from build123d import *

# Parameters (mm, degrees)
SKETCH_W        = 49
SKETCH_H        = 40
PAD_DEPTH       = 33
SKETCH001_W     = 47
SKETCH001_H     = 21
POCKET_DEPTH    = 31
SKETCH002_W     = 42
SKETCH002_H     = 19
POCKET001_DEPTH = 31
SKETCH003_W     = 7
SKETCH003_H     = 7
POCKET002_DEPTH = 31
SKETCH004_W     = 10
SKETCH004_H     = 10
PAD001_DEPTH    = 27
SKETCH005_W     = 10
SKETCH005_H     = 8
POCKET003_DEPTH = 27
SKETCH006_W     = 7
SKETCH006_H     = 12
POCKET004_DEPTH = 4
SKETCH007_W     = 5
SKETCH007_H     = 10
POCKET005_DEPTH = 27
FILLET_R        = 4
SKETCH008_R     = 1.6
POCKET006_DEPTH = 6.001
SKETCH009_R     = 1.6
POCKET007_DEPTH = 6.001
SKETCH010_R     = 2.75
POCKET008_DEPTH = 27
FILLET001_R     = 2
FILLET002_R     = 4
SKETCH011_W     = 11.5
SKETCH011_H     = 8.5
PAD002_DEPTH    = 2
FILLET003_R     = 2
FILLET004_R     = 4
FILLET005_R     = 6
FILLET006_R     = 2
FILLET007_R     = 2


with BuildPart() as part:
    # Sketch → Pad (new body)
    with BuildSketch(Plane.XY):
        with Locations((24.5, 20)):
            Rectangle(SKETCH_W, SKETCH_H)
    extrude(amount=PAD_DEPTH)

    # Sketch001 → Pocket (cut)
    with BuildSketch(Plane.XY):
        with Locations((23.5, 10.5)):
            Rectangle(SKETCH001_W, SKETCH001_H)
    extrude(amount=POCKET_DEPTH, mode=Mode.SUBTRACT)

    # Sketch002 (on Face4 of Pocket) → Pocket001 (cut)
    with BuildSketch(Plane(origin=(0, 0, 0), x_dir=(1, 0, 0), z_dir=(0, 0, -1))):
        with Locations((28, -30.5)):
            Rectangle(SKETCH002_W, SKETCH002_H)
    extrude(amount=-POCKET001_DEPTH, mode=Mode.SUBTRACT)

    # Sketch003 (on Face10 of Pocket001) → Pocket002 (cut)
    with BuildSketch(Plane(origin=(0, 0, 0), x_dir=(1, 0, 0), z_dir=(0, 0, -1))):
        with Locations((3.5, -24.5)):
            Rectangle(SKETCH003_W, SKETCH003_H)
    extrude(amount=-POCKET002_DEPTH, mode=Mode.SUBTRACT)

    # Sketch004 (on Face12 of Pocket002) → Pad001 (join)
    with BuildSketch(Plane(origin=(0, 0, 31), x_dir=(1, 0, 0), z_dir=(0, 0, -1))):
        with Locations((42, -5)):
            Rectangle(SKETCH004_W, SKETCH004_H)
    extrude(amount=PAD001_DEPTH)

    # Sketch005 (on Face7 of Pad001) → Pocket003 (cut)
    with BuildSketch(Plane.XY.offset(33)):
        with Locations((44, 4)):
            Rectangle(SKETCH005_W, SKETCH005_H)
    extrude(amount=-POCKET003_DEPTH, mode=Mode.SUBTRACT)

    # Sketch006 (on Face2 of Pocket003) → Pocket004 (cut)
    with BuildSketch(Plane(origin=(0, 0, 0), x_dir=(1, 0, 0), z_dir=(0, 0, -1))):
        with Locations((3.5, -34)):
            Rectangle(SKETCH006_W, SKETCH006_H)
    extrude(amount=-POCKET004_DEPTH, mode=Mode.SUBTRACT)

    # Sketch007 (on Face7 of Pocket004) → Pocket005 (cut)
    with BuildSketch(Plane.XY.offset(33)):
        with Locations((2.5, 35)):
            Rectangle(SKETCH007_W, SKETCH007_H)
    extrude(amount=-POCKET005_DEPTH, mode=Mode.SUBTRACT)

    # Fillet
    fillet_edges = [part.edges().sort_by_distance(p)[0] for p in [
        (39, 8, 19.5),
    ]]
    fillet(fillet_edges, radius=FILLET_R)

    # Sketch008 (on Face11 of Fillet) → Pocket006 (cut, through all)
    with BuildSketch(Plane.XY.offset(6)):
        with Locations((43, 4)):
            Circle(SKETCH008_R)
    extrude(amount=-POCKET006_DEPTH, mode=Mode.SUBTRACT)

    # Sketch009 (on Face16 of Pocket006) → Pocket007 (cut, through all)
    with BuildSketch(Plane.XY.offset(6)):
        with Locations((3, 36)):
            Circle(SKETCH009_R)
    extrude(amount=-POCKET007_DEPTH, mode=Mode.SUBTRACT)

    # Sketch010 (on Face1 of Pocket007) → Pocket008 (cut)
    with BuildSketch(Plane.XY.offset(33)):
        with Locations((3, 36)):
            Circle(SKETCH010_R)
    extrude(amount=-POCKET008_DEPTH, mode=Mode.SUBTRACT)

    # Fillet001
    fillet001_edges = [part.edges().sort_by_distance(p)[0] for p in [
        (5, 30, 19.5),
    ]]
    fillet(fillet001_edges, radius=FILLET001_R)

    # Fillet002
    fillet002_edges = [part.edges().sort_by_distance(p)[0] for p in [
        (49, 8, 19.5),
    ]]
    fillet(fillet002_edges, radius=FILLET002_R)

    # Sketch011 (on Face5 of Fillet002) → Pad002 (join)
    with BuildSketch(Plane.YZ.offset(49)):
        with Locations((26.75, 26.75)):
            Rectangle(SKETCH011_W, SKETCH011_H)
    extrude(amount=-PAD002_DEPTH)

    # Fillet003
    fillet003_edges = [part.edges().sort_by_distance(p)[0] for p in [
        (48, 21, 22.5),
        (48, 32.5, 31),
    ]]
    fillet(fillet003_edges, radius=FILLET003_R)

    # Fillet004
    fillet004_edges = [part.edges().sort_by_distance(p)[0] for p in [
        (7, 28, 17.5),
    ]]
    fillet(fillet004_edges, radius=FILLET004_R)

    # Fillet005
    fillet005_edges = [part.edges().sort_by_distance(p)[0] for p in [
        (37, 10, 17.5),
    ]]
    fillet(fillet005_edges, radius=FILLET005_R)

    # Fillet006
    fillet006_edges = [part.edges().sort_by_distance(p)[0] for p in [
        (47, 10, 17.5),
    ]]
    fillet(fillet006_edges, radius=FILLET006_R)

    # Fillet007
    fillet007_edges = [part.edges().sort_by_distance(p)[0] for p in [
        (0, 0, 32),
    ]]
    fillet(fillet007_edges, radius=FILLET007_R)


solid = part.part
Check sheet for the modelled part. Datum: model origin and axes. Units: mm. A direction names the side the tool comes from. Coordinates: 2 decimals unless noted, no trailing zeros. Loops run counter-clockwise (first coordinate to the right, second up) from the corner with the lowest first, then second, coordinate; pieces in that order, holes last. Notation, with made-up numbers: (-37, 58) -> (11, 58) arc R14 cw to (11, 73) -> close; hole circle Ø11 at (21.25, 44.25). An arc over 180 degrees is marked (long way). Answer in a Markdown table with one row per item.
1. Release check for a two-part mould opening along X. For faces 5 (the face through (24, 20, 33)), 6 (the face through (49, 20, 17)), 7 (the face through (3.74, 34.58, 5.01)) record: released by +X, released by -X, zero draft, split by the parting line, or undercut.
Check values:
| item | result |
|---|---|
| face 5 | zero draft |
| face 6 | released by +X |
| face 7 | undercut |
2. Sectioned sample at D-D, the plane z = 25. Record the boundary of the cut face in (x, y), then the cut area to 3 significant figures.
Check values:
| item | result |
|---|---|
| outline | (0, 28) -> (3, 28) arc R4 ccw to (7, 32) -> (7, 40) -> (5, 40) -> (5, 37.89) arc R2.75 cw to (5, 34.11) -> (5, 32) arc R2 cw to (3, 30) -> (0, 30) -> close; (37, 0) -> (39, 0) -> (39, 4) arc R4 cw to (43, 8) -> (45, 8) arc R4 ccw to (49, 12) -> (49, 32.5) -> (47, 32.5) -> (47, 12) arc R2 cw to (45, 10) -> (43, 10) arc R6 ccw to (37, 4) -> close |
| area | 108 mm2 |
3. Sectioned sample at A-A, the plane z = 5. Record the boundary of the cut face in (x, y), then the cut area to 3 significant figures.
Check values:
| item | result |
|---|---|
| outline | (0, 28) -> (3, 28) arc R4 ccw to (7, 32) -> (7, 40) -> (0, 40) -> close; (37, 0) -> (49, 0) -> (49, 21) -> (47, 21) -> (47, 12) arc R2 cw to (45, 10) -> (43, 10) arc R6 ccw to (37, 4) -> close; hole circle Ø3.2 at (3, 36); hole circle Ø3.2 at (43, 4) |
| area | 200 mm2 |
4. Go/stop test with flat-tipped pins: pin 1 (3.5 mm diameter, centred on x = 1, z = 17.5, fed in from -Y); pin 2 (3.5 mm diameter, centred on x = 5, y = 36.5, fed in from -Z); pin 3 (2 mm diameter, centred on x = 43.5, z = 13, fed in from -Y). Record where each tip stops, or that it passes through.
Check values:
| item | result |
|---|---|
| pin 1 | stops at y = 28 |
| pin 2 | stops at z = 4 |
| pin 3 | stops at y = 7.97 |
5. Sectioned sample at B-B, the plane z = 9. Record the boundary of the cut face in (x, y), then the cut area to 3 significant figures.
Check values:
| item | result |
|---|---|
| outline | (0, 28) -> (3, 28) arc R4 ccw to (7, 32) -> (7, 40) -> (5, 40) -> (5, 37.89) arc R2.75 cw to (5, 34.11) -> (5, 32) arc R2 cw to (3, 30) -> (0, 30) -> close; (37, 0) -> (39, 0) -> (39, 4) arc R4 cw to (43, 8) -> (45, 8) arc R4 ccw to (49, 12) -> (49, 21) -> (47, 21) -> (47, 12) arc R2 cw to (45, 10) -> (43, 10) arc R6 ccw to (37, 4) -> close |
| area | 84.6 mm2 |
6. Sectioned sample at C-C, the plane y = 36. Record the boundary of the cut face in (x, z).
Check values:
| item | result |
|---|---|
| outline | (0, 4) -> (1.4, 4) -> (1.4, 6) -> (0, 6) -> close; (4.6, 4) -> (7, 4) -> (7, 31) -> (49, 31) -> (49, 33) -> (5.75, 33) -> (5.75, 6) -> (4.6, 6) -> close |
7. Material ranges on line 1 along Z through (x, y) = (26, 22.5); line 2 along X through (y, z) = (14, 12); line 3 along Z through (x, y) = (45.5, 4), recorded low to high. Write a range as [from, to].
Check values:
| item | result |
|---|---|
| line 1 | z = [31, 33] |
| line 2 | x = [47, 49] |
| line 3 | z = [4, 6] |
8. Access from +Z, -Z, +X, -X, +Y, -Y to the whole of each face (thin tool, end or side, straight path). Record for faces 1 (the face through (5.859, 29.203, 17.689)), 2 (the face through (1, 30, 20)), 3 (the face through (38.711, 8.196, 17.311)), 4 (the face through (47.99, 33.1, 30.43)).
Check values:
| item | result |
|---|---|
| face 1 | -Z, -Y |
| face 2 | +Z, -X, +Y |
| face 3 | -Z, -X, +Y |
| face 4 | -Z, +X, +Y |
